Can you work these out from the model? Positions are in its coordinate system, mm. Face numbers are marked on the shaded views. A direction names the side the tool comes from. Give positions to 0.01 mm unless a question says otherwise; leave off trailing zeros. Write each loop counter-clockwise with the first axis right and the second up, starting at its lowest first coordinate (ties: lowest second). Pieces come first, ordered by that corner, then holes.
1. I'm going to push flat-ended pins straight in: pin 1 (1.2 mm diameter, centred on y = 5.5, z = -19.5, fed in from -X); pin 2 (0.6 mm diameter, centred on y = 5.5, z = 0.5, fed in from -X); pin 3 (2 mm diameter, centred on x = 29, y = 2, fed in from +Z). Where does each tip first touch, or does it pass through?
2. On a 3-axis mill with a long thin cutter (end or side, diameter ignored), from which of +Z, -Z, +X, -X, +Y, -Y can I reach the whole of each face in a straight line? I mean the marked faces 4, 5, 6, 7 and 8. Say none if no direction works.
3. If I drill on probe 1 along X at (y, z) = (0.5, -6.25); probe 2 along X at (y, z) = (1.5, -11); probe 3 along Z at (x, y) = (0, 1.25), over which ranges is the centre line in solid material (lowest first)?
4. Suppose I cut it at B-B (x = 0). Please give me the cut outline in (y, z).
5. Thinking about a two-plate mould opening in X: for the marked faces 1, 2 and 3, which applies, pulls with the +X half, pulls with the -X half, needs draft (parallel to the pull), parting line crosses it, or undercut?
6. Suppose I cut it at C-C (z = -8.5). Please give me the cut outline in (x, y).
7. Suppose I cut it at A-A (y = 3.5). Give the number of separate pieces and of enclosed holes in the cut face, and give its area (3 significant figures).
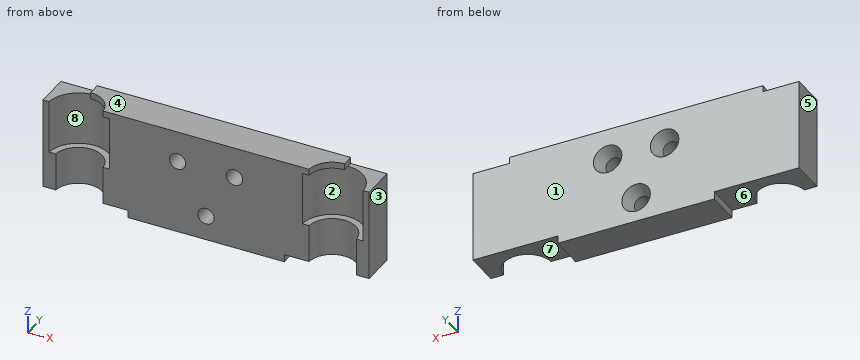
```python
from build123d import *

# Parameters (mm, degrees)
BOSS_EXTRUDE1_DEPTH                               = 7.112
SKETCH2_R                                         = 4.7625
CUT_EXTRUDE1_DEPTH                                = 39.891507997
SKETCH3_R                                         = 6.096
CUT_EXTRUDE2_DEPTH                                = 10.668
CSK_FOR_4_FLAT_HEAD_MACHINE_SCREW_100_D           = 3.2639
CSK_FOR_4_FLAT_HEAD_MACHINE_SCREW_100_CSINK_D     = 5.715
CSK_FOR_4_FLAT_HEAD_MACHINE_SCREW_100_CSINK_ANGLE = 52.893588
BOSS_EXTRUDE2_START                               = 1.27
BOSS_EXTRUDE2_DEPTH                               = 1.27
SKETCH12_W                                        = 65.405
SKETCH12_H                                        = 0.254
CUT_EXTRUDE3_DEPTH                                = 40.553568414


with BuildPart() as part:
    # Sketch1 → Boss-Extrude1 (new body)
    with BuildSketch(Plane(origin=(0, 0, 0), x_dir=(1, 0, 0), z_dir=(0, 1, 0))):
        Polygon((32.7025, 0), (-32.7025, 0), (-32.7025, 18.288), (-15.6845, 18.288), (-15.6845, 19.812), (15.6845, 19.812), (15.6845, 18.288), (32.7025, 18.288), align=None)
    extrude(amount=BOSS_EXTRUDE1_DEPTH)

    # Sketch2 → Cut-Extrude1 (cut, through all)
    with BuildSketch(Plane.XY):
        with Locations((-25.4, -0.1905)):
            Circle(SKETCH2_R)
        with Locations((25.399642811, 0)):
            Circle(SKETCH2_R)
    extrude(amount=-CUT_EXTRUDE1_DEPTH, mode=Mode.SUBTRACT)

    # Sketch3 → Cut-Extrude2 (cut)
    with BuildSketch(Plane.XY):
        with Locations((-25.4, -0.1905)):
            Circle(SKETCH3_R)
        with Locations((25.399642811, 0)):
            Circle(SKETCH3_R)
    extrude(amount=-CUT_EXTRUDE2_DEPTH, mode=Mode.SUBTRACT)

    # CSK for #4 Flat Head Machine Screw (100)1 (through all)
    with Locations(Plane(origin=(0, 7.112, 0), x_dir=(1, 0, 0), z_dir=(0, 1, 0))):
        with Locations((0, 14.855335183), (-5.715, 4.956664817), (5.715, 4.956664817)):
            CounterSinkHole(CSK_FOR_4_FLAT_HEAD_MACHINE_SCREW_100_D / 2, CSK_FOR_4_FLAT_HEAD_MACHINE_SCREW_100_CSINK_D / 2, counter_sink_angle=CSK_FOR_4_FLAT_HEAD_MACHINE_SCREW_100_CSINK_ANGLE)

    # Sketch11 → Boss-Extrude2 (add)
    with BuildSketch(Plane.XY.offset(BOSS_EXTRUDE2_START)):
        with BuildLine():
            Line((-20.641311525, 0), (20.637142811, 0))
            ThreePointArc((20.637142811, 0), (22.032046766, 3.367596045), (25.399642811, 4.7625))
            Line((25.399642811, 4.7625), (25.399642811, 7.112))
            Line((25.399642811, 7.112), (-25.4, 7.112))
            Line((-25.4, 7.112), (-25.4, 4.572))
            ThreePointArc((-25.4, 4.572), (-22.100443212, 3.24378759), (-20.641311525, 0))
        make_face()
    extrude(amount=-BOSS_EXTRUDE2_DEPTH)

    # Sketch12 → Cut-Extrude3 (cut, through all)
    with BuildSketch(Plane(origin=(0, 0, -19.812), x_dir=(-1, 0, 0), z_dir=(0, 0, -1))):
        with Locations((0, 0.127)):
            Rectangle(SKETCH12_W, SKETCH12_H)
    extrude(amount=-CUT_EXTRUDE3_DEPTH, mode=Mode.SUBTRACT)


solid = part.part
```
Checks:
1. pin 1: stops at x = -15.68
1. pin 2: stops at x = -25.4
1. pin 3: stops at z = -10.67
2. face 4: +Z, +X, -X, +Y, -Y
2. face 5: +Z, -Z, -X, +Y, -Y
2. face 6: -Z, -X, +Y, -Y
2. face 7: -Z, +X, +Y, -Y
2. face 8: -Y
3. probe 1: x = -32.7 to -31.46, -19.34 to -6.71, -4.72 to 4.72, 6.71 to 19.32, 31.48 to 32.7
3. probe 2: x = -32.7 to -29.85, -20.95 to 20.88, 29.92 to 32.7
3. probe 3: z = -19.81 to -16.49, -13.22 to 1.27
4. outline: (0.25, -19.81) - (7.11, -19.81) - (7.11, -17.71) - (4.65, -16.49) - (0.25, -16.49) - close; (0.25, -13.22) - (4.65, -13.22) - (7.11, -12) - (7.11, 1.27) - (0.25, 1.27) - close
5. face 1: needs draft
5. face 2: undercut
5. face 3: pulls with the +X half
6. outline: (-32.7, 0.25) - (-31.48, 0.25) arc R6.1 cw to (-19.32, 0.25) - (19.31, 0.25) arc R6.1 cw to (31.49, 0.25) - (32.7, 0.25) - (32.7, 7.11) - (-32.7, 7.11) - close
7. separate pieces: 3
7. enclosed holes: 3
7. area: 970 mm2
